Part print with two shaded views. Sizes in mm from the minimum x, y, z corner. Round coordinates to 2 decimals unless told otherwise and drop trailing zeros. Write each loop counter-clockwise with the first axis right and the second up, starting at its lowest first coordinate (ties: lowest second). Pieces come first, ordered by that corner, then holes. Notation, with made-up numbers: M 69.5,35.5 L 88.5,35.5 A22 cw 88.5,47.5 Z; hole C 3.5,71 d2. An arc over 180 degrees is marked long. One line per question, with ' | ' between items. Start each with the question number.
1) Drop flat-ended pins along their axis: pin 1 Ø8 at (x, y) = (31, 39) entering from -Z; pin 2 Ø4 at (y, z) = (39.5, 8.5) entering from +X; pin 3 Ø12 at (x, z) = (65, 14) entering from +Y; pin 4 Ø12 at (y, z) = (56.5, 9) entering from -X. Give the stop position or say it passes through.
2) Mould opens along X. For the marked faces 1 and 2 say: pulls with the +X half, pulls with the -X half, needs draft (parallel to the pull), parting line crosses it, or undercut.
3) Saw through at B-B (x = 15). List the corners of the cut face in (y, z).
4) Saw through at D-D (z = 8.75). List the corners of the cut face in (x, y), plus the area to 3 significant figures.
5) Wall check: probe 1 along X at (y, z) = (15, 18.5); probe 2 along X at (y, z) = (52.5, 8); probe 3 along X at (y, z) = (11, 12) (1 decimal). Give the ranges that are in metal, low to high. Write a range as [from, to].
6) Saw through at A-A (y = 52.5). List the corners of the cut face in (x, z).
7) Saw through at C-C (y = 15). List the corners of the cut face in (x, z).
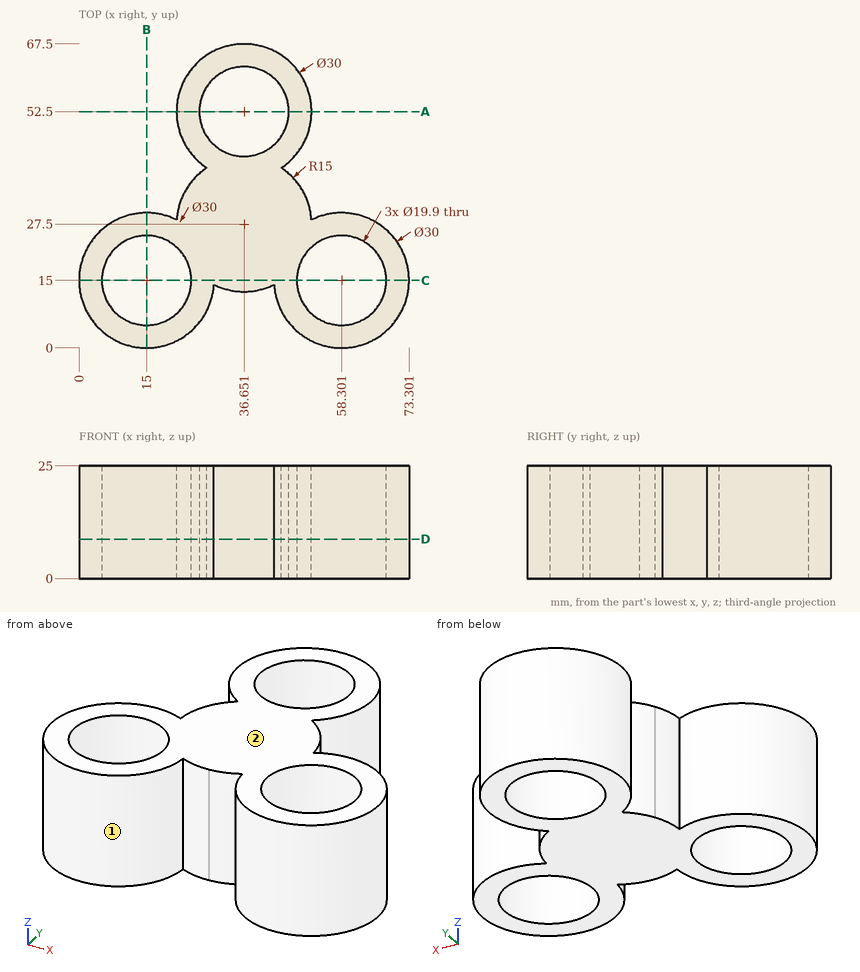
Answer key:
1) pin 1: stops at z = 0 | pin 2: stops at x = 47.83 | pin 3: stops at y = 29.98 | pin 4: stops at x = 21.65
2) face 1: undercut | face 2: needs draft
3) outline: M 0,0 L 5.05,0 L 5.05,25 L 0,25 Z; M 24.95,0 L 30,0 L 30,25 L 24.95,25 Z
4) outline: M 21.68,28.43 A15 ccw long 29.97,14.07 A15 ccw 36.65,12.5 A15 ccw 43.33,14.07 A15 ccw long 51.62,28.43 A15 ccw 49.64,35 A15 ccw 44.94,40 A15 ccw long 28.36,40 A15 ccw 23.66,35 A15 ccw Z; hole C 15,15 d19.9; hole C 36.65,52.5 d19.9; hole C 58.3,15 d19.9 | area: 1,730 mm2
5) probe 1: x = [0, 5.05], [24.95, 48.35], [68.25, 73.3] | probe 2: x = [21.65, 26.7], [46.6, 51.65] | probe 3: x = [0.5, 5.9], [24.1, 29.5], [43.8, 49.2], [67.4, 72.8]
6) outline: M 21.65,0 L 26.7,0 L 26.7,25 L 21.65,25 Z; M 46.6,0 L 51.65,0 L 51.65,25 L 46.6,25 Z
7) outline: M 0,0 L 5.05,0 L 5.05,25 L 0,25 Z; M 24.95,0 L 48.35,0 L 48.35,25 L 24.95,25 Z; M 68.25,0 L 73.3,0 L 73.3,25 L 68.25,25 Z
